For this review, take the finished solid that the model builds, in its own axes (mm). A direction names the side the tool comes from. Coordinates: 2 decimals unless noted, no trailing zeros. Loops run counter-clockwise (first coordinate to the right, second up) from the corner with the lowest first, then second, coordinate; pieces in that order, holes last. Notation, with made-up numbers: (43.5, 8) - (96.5, 8) arc R21 cw to (96.5, 27) - close; hole circle Ø6 at (68, 7). An arc over 180 degrees is marked (long way). One line per item, written item: value. Start each with the question number.
1. For faces 4 (the face through (-35, -1, 0)), 5 (the face through (-0.793, 55.859, -36.077)), 6 (the face through (-0.793, -56.155, -36.077)), list the 3-axis set-ups (+Z, -Z, +X, -X, +Y, -Y) from which the entire face can be reached by the end or side of a thin tool; tool diameter is ignored.
2. Insertion check: pin 1 (15.5 mm diameter, centred on x = 48.15, y = 0, fed in from -Z); pin 2 (2 mm diameter, centred on x = -28.5, z = -40.5, fed in from -Y). Each pin has a flat end and moves straight along its axis. Give the tip position at first contact, or say it passes through.
3. The part is to be moulded in two halves that separate along X. For faces 1 (the face through (63.451, -1, -35)), 2 (the face through (34, -1, 0)), 3 (the face through (-0.51, -0.932, -23.202)), say which applies: released by +X, released by -X, zero draft, split by the parting line, or undercut.
4. Take a section at C-C, the plane x = 0. State the section outline as (y, z) points.
5. Take a section at D-D, the plane z = -53.5. State the section outline as (x, y) points.
6. Take a section at A-A, the plane y = 0. State the section outline as (x, z) points.
7. To check wall thickness, follow line 1 (X direction, y = 0, z = -42.5); line 2 (X direction, y = 2.5, z = -58.5); line 3 (X direction, y = 9, z = -19.5). State the ranges of each line that lie inside material, in increasing order. Write a range as from..to.
8. Take a section at B-B, the plane z = -7. State the section outline as (x, y) points.
```python
from build123d import *

# Parameters (mm, degrees)
F0_W     = 126.902834
F0_H     = 138.312936
F1_DEPTH = 45.466
F2_R     = 36.085461
F3_DEPTH = 66.548
F4_R     = 23.207671
F5_DEPTH = 157.988
F6_W     = 174.213074
F6_H     = 78.061931
F7_DEPTH = 75.946
F8_R     = 9.741343
F9_DEPTH = 80.264


with BuildPart() as f1:
    # F0 (on Front) → F1 (new body, symmetric)
    with BuildSketch(Plane.XZ):
        Rectangle(F0_W, F0_H)
    extrude(amount=F1_DEPTH, both=True)

    # F2 (on Front) → F3 (join, symmetric)
    with BuildSketch(Plane.XZ):
        Circle(F2_R)
    extrude(amount=F3_DEPTH, both=True)

    # F4 (on face) → F5 (cut)
    with BuildSketch(Plane.XZ.offset(66.548)):
        Circle(F4_R)
    extrude(amount=-F5_DEPTH, mode=Mode.SUBTRACT)

    # F6 (on Front) → F7 (cut, symmetric)
    with BuildSketch(Plane.XZ):
        with Locations((2.504658, 39.030966)):
            Rectangle(F6_W, F6_H)
    extrude(amount=F7_DEPTH, both=True, mode=Mode.SUBTRACT)

    # F8 (on face) → F9 (cut)
    with BuildSketch(Plane(origin=(0, 0, -69.156468), x_dir=(1, 0, 0), z_dir=(0, 0, -1))):
        with Locations((48.145149, 0)):
            Circle(F8_R)
        with Locations((-48.145149, 0)):
            Circle(F8_R)
    extrude(amount=-F9_DEPTH, mode=Mode.SUBTRACT)


solid = f1.part
```
Solutions:
1. face 4: +Z, +X, -X, +Y, -Y
1. face 5: -Z, +Y
1. face 6: -Z, -Y
2. pin 1: through
2. pin 2: y = -45.47
3. face 1: released by +X
3. face 2: zero draft
3. face 3: undercut
4. outline: (-66.55, -36.09) - (-45.47, -36.09) - (-45.47, -69.16) - (45.47, -69.16) - (45.47, -36.09) - (66.55, -36.09) - (66.55, -23.21) - (-66.55, -23.21) - close
5. outline: (-63.45, -45.47) - (63.45, -45.47) - (63.45, 45.47) - (-63.45, 45.47) - close; hole circle Ø19.48 at (-48.15, 0); hole circle Ø19.48 at (48.15, 0)
6. outline: (-63.45, -69.16) - (-57.89, -69.16) - (-57.89, 0) - (-63.45, 0) - close; (-38.4, -69.16) - (38.4, -69.16) - (38.4, 0) - (23.21, 0) arc R23.21 cw to (-23.21, 0) - (-38.4, 0) - close; (57.89, -69.16) - (63.45, -69.16) - (63.45, 0) - (57.89, 0) - close
7. line 1: -63.45..-57.89, -38.4..38.4, 57.89..63.45
7. line 2: -63.45..-57.56, -38.73..38.73, 57.56..63.45
7. line 3: -63.45..-51.87, -44.42..-12.58, 12.58..44.42, 51.87..63.45
8. outline: (-63.45, -45.47) - (-35.4, -45.47) - (-35.4, -66.55) - (-22.13, -66.55) - (-22.13, 66.55) - (-35.4, 66.55) - (-35.4, 45.47) - (-63.45, 45.47) - close; (22.13, -66.55) - (35.4, -66.55) - (35.4, -45.47) - (63.45, -45.47) - (63.45, 45.47) - (35.4, 45.47) - (35.4, 66.55) - (22.13, 66.55) - close; hole circle Ø19.48 at (-48.15, 0); hole circle Ø19.48 at (48.15, 0)
